Verification items for the finished model (mm, model axes). A direction names the side the tool comes from. Round coordinates to 2 decimals unless told otherwise and drop trailing zeros. Write each loop counter-clockwise with the first axis right and the second up, starting at its lowest first coordinate (ties: lowest second). Pieces come first, ordered by that corner, then holes. Notation, with made-up numbers: M -22,33.25 L 23,33.25 A26 cw 23,55.25 Z; hole C 27.5,35 d1. An arc over 180 degrees is marked long. One line per item, written item: value. Start each with the question number.
Item 1: Draft check along X on faces 4 (the face through (0, 3, -113)), 5 (the face through (254, 3, -113)), 6 (the face through (6.969, 3.885, -131.957)). Enter one of: +X half, -X half, draft (parallel to the pull), parting line (faces both ways), or undercut.
Item 2: Section check D-D, the plane y = 4.5. State how many separate pieces and enclosed holes the cut face has, then the cut area to 3 significant figures.
Item 3: Gauge pin test, flat ends, axial feed: pin 1 (2 mm diameter, centred on y = 2.5, z = -75, fed in from -X); pin 2 (4.5 mm diameter, centred on x = 246.38, z = -127, fed in from -Y); pin 3 (3 mm diameter, centred on x = 249, z = -128, fed in from +Y). Record the tip position at first contact, or that the pin passes through.
Item 4: Section check B-B, the plane x = 121.5. Record the cut outline in (y, z).
Item 5: Thickness scan on probe 1 along Z at (x, y) = (49.5, 2.75); probe 2 along X at (y, z) = (4.1, -76.2); probe 3 along Z at (x, y) = (7.62, 2.8). Record the ranges inside material, lowest first. Write a range as from..to.
Item 6: Section check A-A, the plane z = -108. Record the cut outline in (x, y), then the cut area to 3 significant figures.
Item 7: Section check C-C, the plane z = -12.7. Record the cut outline in (x, y), then the cut area to 3 significant figures.
Item 8: Tool access check on faces 1 (the face through (126, 3, -177.8)), 2 (the face through (125, 3, -222.25)), 3 (the face through (8.02, 4.87, -16.99)). Record the directions out of +Z, -Z, +X, -X, +Y, -Y that give a thin tool (end or side, any length) a straight path to the whole face; none if there is none.
from build123d import *

# Parameters (mm, degrees)
SKETCH1_W                      = 254
SKETCH1_H                      = 203.2
SKETCH1_R                      = 3.05
SKETCH1_W_2                    = 203.2
SKETCH1_H_2                    = 152.4
BOSS_EXTRUDE1_DEPTH            = 6.35
SKETCH2_R                      = 6.35
CUT_EXTRUDE1_DEPTH             = 3
CBORE_FOR_M5_SHCS1_D           = 5.499989
CBORE_FOR_M5_SHCS1_CBORE_D     = 10
CBORE_FOR_M5_SHCS1_CBORE_DEPTH = 5
SKETCH5_W                      = 254
SKETCH5_H                      = 19.05
BOSS_EXTRUDE3_DEPTH            = 6.35
SKETCH6_R                      = 2
CUT_EXTRUDE2_DEPTH             = 4.5
SKETCH7_R                      = 1.75
CUT_EXTRUDE3_DEPTH             = 4.5


with BuildPart() as part:
    # Sketch1 → Boss-Extrude1 (new body)
    with BuildSketch(Plane(origin=(0, 0, 0), x_dir=(1, 0, 0), z_dir=(0, 1, 0))):
        with Locations((127, 101.6)):
            Rectangle(SKETCH1_W, SKETCH1_H)
        with Locations((12.7, 190.5)):
            Circle(SKETCH1_R, mode=Mode.SUBTRACT)
        with Locations((241.3, 190.5)):
            Circle(SKETCH1_R, mode=Mode.SUBTRACT)
        with Locations((241.3, 12.7)):
            Circle(SKETCH1_R, mode=Mode.SUBTRACT)
        with Locations((12.7, 12.7)):
            Circle(SKETCH1_R, mode=Mode.SUBTRACT)
        with Locations((127, 101.6)):
            Rectangle(SKETCH1_W_2, SKETCH1_H_2, mode=Mode.SUBTRACT)
    extrude(amount=BOSS_EXTRUDE1_DEPTH)

    # Sketch2 → Cut-Extrude1 (cut)
    with BuildSketch(Plane(origin=(0, 6.35, 0), x_dir=(1, 0, 0), z_dir=(0, 1, 0))):
        with Locations((12.7, 190.5)):
            Circle(SKETCH2_R)
        with Locations((241.3, 190.5)):
            Circle(SKETCH2_R)
        with Locations((241.3, 12.7)):
            Circle(SKETCH2_R)
        with Locations((12.7, 12.7)):
            Circle(SKETCH2_R)
    extrude(amount=-CUT_EXTRUDE1_DEPTH, mode=Mode.SUBTRACT)

    # CBORE for M5 SHCS1 (through all)
    with Locations(Plane(origin=(0, 6.35, 0), x_dir=(1, 0, 0), z_dir=(0, 1, 0))):
        with Locations((246.38, 76.2), (246.38, 127), (7.62, 76.2), (7.62, 127)):
            CounterBoreHole(CBORE_FOR_M5_SHCS1_D / 2, CBORE_FOR_M5_SHCS1_CBORE_D / 2, CBORE_FOR_M5_SHCS1_CBORE_DEPTH)

    # Sketch5 → Boss-Extrude3 (add)
    with BuildSketch(Plane.XZ):
        with Locations((127, -212.725)):
            Rectangle(SKETCH5_W, SKETCH5_H)
    extrude(amount=-BOSS_EXTRUDE3_DEPTH)

    # Sketch6 → Cut-Extrude2 (cut)
    with BuildSketch(Plane(origin=(0, 6.35, 0), x_dir=(1, 0, 0), z_dir=(0, 1, 0))):
        with Locations((19.924999942, 216.120415829)):
            Circle(SKETCH6_R)
        with Locations((34.924999942, 216.120415829)):
            Circle(SKETCH6_R)
        with Locations((49.936813619, 216.120415829)):
            Circle(SKETCH6_R)
        with Locations((204.063186381, 216.120415829)):
            Circle(SKETCH6_R)
        with Locations((219.075000058, 216.120415829)):
            Circle(SKETCH6_R)
        with Locations((234.075000058, 216.120415829)):
            Circle(SKETCH6_R)
    extrude(amount=-CUT_EXTRUDE2_DEPTH, mode=Mode.SUBTRACT)

    # Sketch7 → Cut-Extrude3 (cut)
    with BuildSketch(Plane(origin=(0, 1.85, 0), x_dir=(1, 0, 0), z_dir=(0, 1, 0))):
        with Locations((19.924999942, 216.120415829)):
            Circle(SKETCH7_R)
        with Locations((34.924999942, 216.120415829)):
            Circle(SKETCH7_R)
        with Locations((49.936813619, 216.120415829)):
            Circle(SKETCH7_R)
        with Locations((204.063186381, 216.120415829)):
            Circle(SKETCH7_R)
        with Locations((219.075000058, 216.120415829)):
            Circle(SKETCH7_R)
        with Locations((234.075000058, 216.120415829)):
            Circle(SKETCH7_R)
    extrude(amount=-CUT_EXTRUDE3_DEPTH, mode=Mode.SUBTRACT)


solid = part.part
Response values:
1. face 4: -X half
1. face 5: +X half
1. face 6: undercut
2. separate pieces: 1
2. enclosed holes: 15
2. area: 24,600 mm2
3. pin 1: stops at x = 0
3. pin 2: passes through
3. pin 3: stops at y = 1.35
4. outline: M 0,-222.25 L 6.35,-222.25 L 6.35,-177.8 L 0,-177.8 Z; M 0,-25.4 L 6.35,-25.4 L 6.35,0 L 0,0 Z
5. probe 1: z = -222.25..-218.07, -214.17..-177.8, -25.4..0
5. probe 2: x = 0..2.62, 12.62..25.4, 228.6..241.38, 251.38..254
5. probe 3: z = -222.25..-132, -122..-81.2, -71.2..0
6. outline: M 0,0 L 25.4,0 L 25.4,6.35 L 0,6.35 Z; M 228.6,0 L 254,0 L 254,6.35 L 228.6,6.35 Z
6. area: 323 mm2
7. outline: M 0,0 L 9.65,0 L 9.65,3.35 L 6.35,3.35 L 6.35,6.35 L 0,6.35 Z; M 15.75,0 L 238.25,0 L 238.25,3.35 L 234.95,3.35 L 234.95,6.35 L 19.05,6.35 L 19.05,3.35 L 15.75,3.35 Z; M 244.35,0 L 254,0 L 254,6.35 L 247.65,6.35 L 247.65,3.35 L 244.35,3.35 Z
7. area: 1,500 mm2
8. face 1: +Y, -Y
8. face 2: -Z, +X, -X, +Y, -Y
8. face 3: +Y
